Geometry: final body of the model. Coordinates: model frame, mm. Face numbers are marked on the shaded views. A direction names the side the tool comes from. Give positions to 0.01 mm unless a question says otherwise; leave off trailing zeros. Order: outer loops, then holes, each group sorted by start corner. A loop starts at its lowest first (then second) coordinate and runs counter-clockwise, first axis right, second up. Notation, with made-up numbers: (45.25, 58.5) -> (77.25, 58.5) arc R10 ccw to (77.25, 67.5) -> close; hole circle Ø8 at (-22.5, 81.5). An arc over 180 degrees is marked (long way). One line per item, written item: value. Start each with the question number.
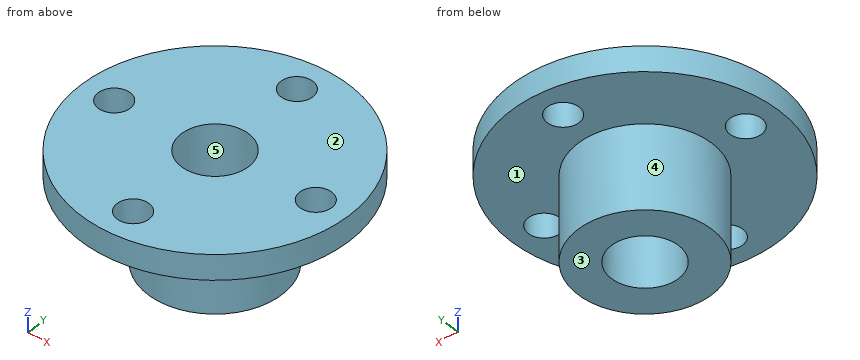
```python
from build123d import *

# Parameters (mm, degrees)
SKETCH1_R           = 15.9
BOSS_EXTRUDE1_DEPTH = 3
SKETCH2_R           = 7.95
BOSS_EXTRUDE2_DEPTH = 10
SKETCH3_R           = 4
CUT_EXTRUDE1_DEPTH  = 20
SKETCH4_R           = 1.9
CUT_EXTRUDE2_DEPTH  = 20


with BuildPart() as part:
    # Sketch1 → Boss-Extrude1 (new body)
    with BuildSketch(Plane.XY):
        Circle(SKETCH1_R)
    extrude(amount=BOSS_EXTRUDE1_DEPTH)

    # Sketch2 → Boss-Extrude2 (add)
    with BuildSketch(Plane(origin=(0, 0, 0), x_dir=(-1, 0, 0), z_dir=(0, 0, -1))):
        Circle(SKETCH2_R)
    extrude(amount=BOSS_EXTRUDE2_DEPTH)

    # Sketch3 → Cut-Extrude1 (cut)
    with BuildSketch(Plane(origin=(0, 0, -10), x_dir=(-1, 0, 0), z_dir=(0, 0, -1))):
        Circle(SKETCH3_R)
    extrude(amount=-CUT_EXTRUDE1_DEPTH, mode=Mode.SUBTRACT)

    # Sketch4 → Cut-Extrude2 (cut)
    with BuildSketch(Plane(origin=(0, 0, 0), x_dir=(-1, 0, 0), z_dir=(0, 0, -1))):
        with Locations((0, 12)):
            Circle(SKETCH4_R)
        with Locations((-12, 0)):
            Circle(SKETCH4_R)
        with Locations((12, 0)):
            Circle(SKETCH4_R)
        with Locations((0, -12)):
            Circle(SKETCH4_R)
    extrude(amount=-CUT_EXTRUDE2_DEPTH, mode=Mode.SUBTRACT)


solid = part.part
```
1. Pin query (flat end, axial travel): P1, Ø2, axis at x = 5.5, z = -2.5, coming from the +Y side; P2, Ø1.5, axis at y = -3, z = -0.5, coming from the +X side; P3, Ø5, axis at y = -6, z = -5.5, coming from the -X side; P4, Ø6, axis at y = -0.5, z = -1.5, coming from the +X side. Return the tip coordinate at first contact, or that it passes through.
2. Access query for the marked faces 1 and 2. Directions: +Z, -Z, +X, -X, +Y, -Y. A direction counts if a zero-diameter tool reaches every point of the face in a straight line with its end or side. Return the directions, or none.
3. Cut plane A-A, the plane y = 0. Return loops of the section in (x, z).
4. Cut plane C-C, the plane y = 13. Return loops of the section in (x, z), then the cut area to 3 significant figures.
5. Draft query along Y for the marked faces 3, 4 and 5. Return one class per face: pulls with the +Y half, pulls with the -Y half, needs draft (parallel to the pull), parting line crosses it, or undercut.
6. Cut plane D-D, the plane x = 11.5. Return loops of the section in (y, z), then the cut area to 3 significant figures.
7. Material intervals for L1, parallel to Y at x = 0, z = 1.5; L2, parallel to Y at x = 0, z = -1.5; L3, parallel to Z at x = 8.5, y = 2, sorted ascending. Write a range as [from, to].
Answers follow:
1. P1: stops at y = 6.55
1. P2: stops at x = 15.71
1. P3: stops at x = -7.14
1. P4: stops at x = 15.9
2. face 1: -Z
2. face 2: +Z, +X, -X, +Y, -Y
3. outline: (-15.9, 0) -> (-13.9, 0) -> (-13.9, 3) -> (-15.9, 3) -> close; (-10.1, 0) -> (-7.95, 0) -> (-7.95, -10) -> (-4, -10) -> (-4, 3) -> (-10.1, 3) -> close; (4, -10) -> (7.95, -10) -> (7.95, 0) -> (10.1, 0) -> (10.1, 3) -> (4, 3) -> close; (13.9, 0) -> (15.9, 0) -> (15.9, 3) -> (13.9, 3) -> close
4. outline: (-9.15, 0) -> (-1.62, 0) -> (-1.62, 3) -> (-9.15, 3) -> close; (1.62, 0) -> (9.15, 0) -> (9.15, 3) -> (1.62, 3) -> close
4. area: 45.2 mm²
5. face 3: needs draft
5. face 4: parting line crosses it
5. face 5: undercut
6. outline: (-10.98, 0) -> (-1.83, 0) -> (-1.83, 3) -> (-10.98, 3) -> close; (1.83, 0) -> (10.98, 0) -> (10.98, 3) -> (1.83, 3) -> close
6. area: 54.9 mm²
7. L1: y = [-15.9, -13.9], [-10.1, -4], [4, 10.1], [13.9, 15.9]
7. L2: y = [-7.95, -4], [4, 7.95]
7. L3: z = [0, 3]
